Autodesk Inventor part; units mm, degrees
ref_plane "YZ Plane" through (0, 0, 0) normal (1, 0, 0) x (0, 1, 0)
ref_plane "XZ Plane" through (0, 0, 0) normal (0, 1, 0) x (-1, 0, 0)
ref_plane "XY Plane" through (0, 0, 0) normal (0, 0, 1) x (1, 0, 0)
sketch "Sketch1" plane through (0, 0, 0) normal (0, 0, 1) x (1, 0, 0)
  line L0 (-45, -30) -> (45, -30)
  line L1 (45, -30) -> (45, 30)
  line L2 (45, 30) -> (-45, 30)
  line L3 (-45, 30) -> (-45, -30)
  line L4 (-45, -30) -> (45, 30) construction
  line L5 (45, -30) -> (-45, 30) construction
  circle A0 centre (-35, -28) radius 1.092
  circle A1 centre (35, -20) radius 1.092
  line L6 (0, 0) -> (14.1537, 0) construction
  circle A2 centre (-35, 28) radius 1.092
  circle A3 centre (35, 20) radius 1.092
  circle A4 centre (-20, 10) radius 1.5
  circle A5 centre (0, 10) radius 1.5
  circle A6 centre (20, 10) radius 1.5
  circle A7 centre (-20, -10) radius 1.5
  circle A8 centre (0, -10) radius 1.5
  circle A9 centre (20, -10) radius 1.5
  dimension "d0" = 90
  dimension "d1" = 60
  dimension "d7" = 2.184
  dimension "d8" = 2.184
  dimension "d11" = 2
  dimension "d19" = 70
  dimension "d22" = 10
  dimension "d23" = 10
  dimension "d24" = 3
  dimension "d25" = 3
  dimension "d26" = 3
  dimension "d27" = 3
  dimension "d28" = 3
  dimension "d29" = 3
  dimension "d30" = 10
  dimension "d31" = 10
  dimension "d32" = 20
  dimension "d33" = 20
extrude "Extrusion1" add sketch "Sketch1" along normal blind 5.1
properties part number "lidar mounting plate"
Verification items for the finished model (mm, model axes). Give positions to 0.01 mm unless a question says otherwise; leave off trailing zeros. Order: outer loops, then holes, each group sorted by start corner. A loop starts at its lowest first (then second) coordinate and runs counter-clockwise, first axis right, second up. Notation, with made-up numbers: M -20.5,58 L 30.5,58 A7 ccw 30.5,62 Z; hole C 80.5,53 d11. An arc over 180 degrees is marked long. Answer as a JSON object with one key per item and string values. Group by question number.
1) Scan lines: line 1 along Y through (x, z) = (-20, 2.7); line 2 along X through (y, z) = (19.5, 2.85). Record each from-to range of solid material in increasing order. Write a range as [from, to].
2) Depth check by flat-ended pin: pin 1 Ø3 at (x, y) = (22.5, 9.5) entering from -Z. Enter the tip coordinate at first touch or a pass-through.
3) Mould release check, pull along Y, two halves, no side actions. Record for faces 1 (the face through (-1, 0, 5.1)), 2 (the face through (1, 30, 3)), 3 (the face through (18.5, -10.07, 2.51)): released by +Y, released by -Y, zero draft, split by the parting line, or undercut.
4) Cross-section at D-D (x = 20). Enter the section's corners in (y, z).
5) Cross-section at B-B (y = -10). Enter the section's corners in (x, z), then the cut area to 3 significant figures.
6) Cross-section at A-A (x = 35). Enter the section's corners in (y, z).
7) Cross-section at C-C (y = 20). Enter the section's corners in (x, z), then the cut area to 3 significant figures.
Result sheet:
{
 "1": {"line 1": "y = [-30, -11.5], [-8.5, 8.5], [11.5, 30]", "line 2": "x = [-45, 34.03], [35.97, 45]"},
 "2": {"pin 1": "stops at z = 0"},
 "3": {"face 1": "zero draft", "face 2": "released by +Y", "face 3": "undercut"},
 "4": {"outline": "M -30,0 L -11.5,0 L -11.5,5.1 L -30,5.1 Z; M -8.5,0 L 8.5,0 L 8.5,5.1 L -8.5,5.1 Z; M 11.5,0 L 30,0 L 30,5.1 L 11.5,5.1 Z"},
 "5": {"outline": "M -45,0 L -21.5,0 L -21.5,5.1 L -45,5.1 Z; M -18.5,0 L -1.5,0 L -1.5,5.1 L -18.5,5.1 Z; M 1.5,0 L 18.5,0 L 18.5,5.1 L 1.5,5.1 Z; M 21.5,0 L 45,0 L 45,5.1 L 21.5,5.1 Z", "area": "413 mm2"},
 "6": {"outline": "M -30,0 L -21.09,0 L -21.09,5.1 L -30,5.1 Z; M -18.91,0 L 18.91,0 L 18.91,5.1 L -18.91,5.1 Z; M 21.09,0 L 30,0 L 30,5.1 L 21.09,5.1 Z"},
 "7": {"outline": "M -45,0 L 33.91,0 L 33.91,5.1 L -45,5.1 Z; M 36.09,0 L 45,0 L 45,5.1 L 36.09,5.1 Z", "area": "448 mm2"}
}
